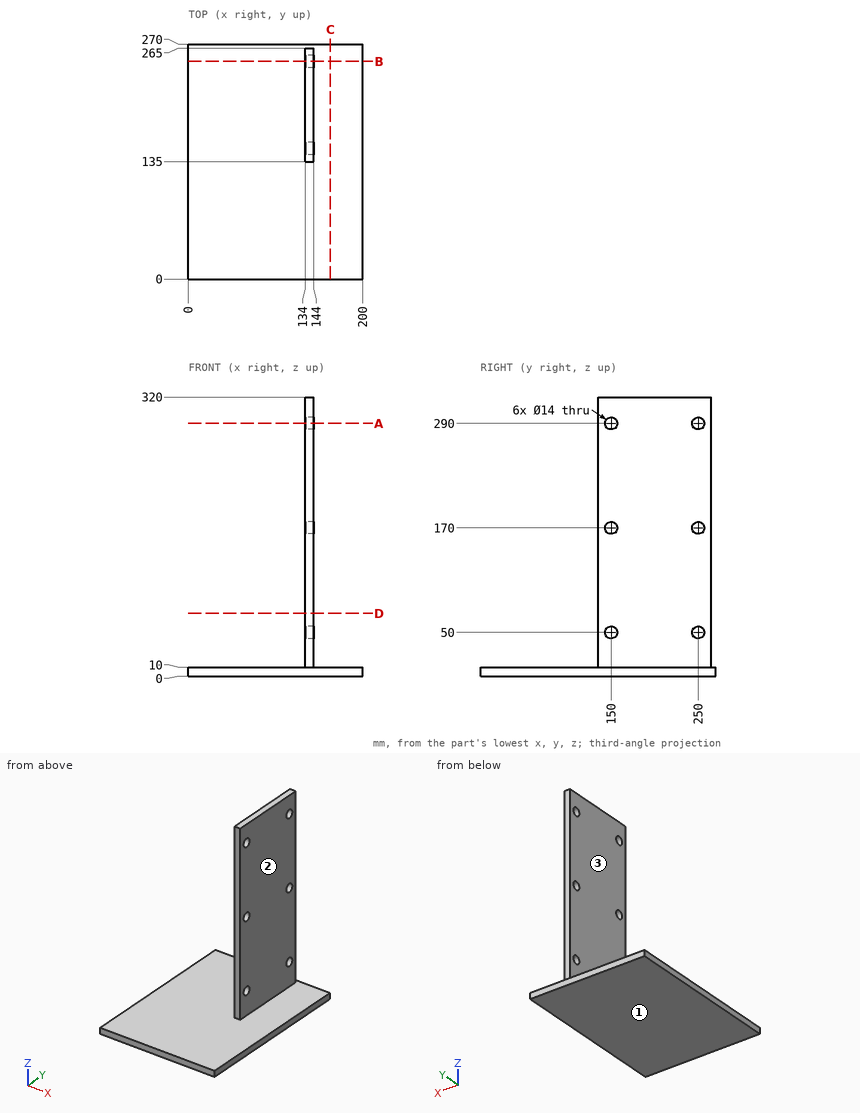
Check sheet for the drawn part. Datum: minimum x, y, z corner. Units: mm. A direction names the side the tool comes from. Round coordinates to 2 decimals unless told otherwise and drop trailing zeros. Write each loop counter-clockwise with the first axis right and the second up, starting at its lowest first coordinate (ties: lowest second). Pieces come first, ordered by that corner, then holes. Notation, with made-up numbers: (28.5, 83) -> (65.5, 83) arc R7 ccw to (65.5, 96) -> close; hole circle Ø8 at (86.25, -35). An arc over 180 degrees is marked (long way). One line per item, written item: value. Start each with the question number.
(1) Go/stop test with flat-tipped pins: pin 1 Ø8.5 at (y, z) = (150, 170) entering from -X; pin 2 Ø22.5 at (y, z) = (150, 50) entering from -X; pin 3 Ø10 at (x, y) = (64, 67) entering from +Z; pin 4 Ø8 at (x, z) = (137.5, 172.5) entering from -Y. Record where each tip stops, or that it passes through.
(2) Cross-section at A-A, the plane z = 290. Record the cut outline in (x, y).
(3) Scan lines: line 1 (Z direction, x = 139.25, y = 250); line 2 (Z direction, x = 109, y = 100); line 3 (X direction, y = 246, z = 143). Record each from-to range of solid material in increasing order. Write a range as [from, to].
(4) Access from +Z, -Z, +X, -X, +Y, -Y to the whole of each face (thin tool, end or side, straight path). Record for the marked faces 1, 2 and 3.
(5) Cross-section at D-D, the plane z = 72. Record the cut outline in (x, y).
(6) Cross-section at B-B, the plane y = 250. Record the cut outline in (x, z), and give its area (3 significant figures).
(7) Cross-section at C-C, the plane x = 163. Record the cut outline in (y, z).
Answer:
1. pin 1: through
1. pin 2: x = 134
1. pin 3: z = 10
1. pin 4: y = 135
2. outline: (134, 135) -> (144, 135) -> (144, 143) -> (134, 143) -> close; (134, 157) -> (144, 157) -> (144, 243) -> (134, 243) -> close; (134, 257) -> (144, 257) -> (144, 265) -> (134, 265) -> close
3. line 1: [0, 43], [57, 163], [177, 283], [297, 320]
3. line 2: [0, 10]
3. line 3: [134, 144]
4. face 1: -Z, +X, -X, +Y, -Y
4. face 2: +Z, +X, +Y, -Y
4. face 3: +Z, -X, +Y, -Y
5. outline: (134, 135) -> (144, 135) -> (144, 265) -> (134, 265) -> close
6. outline: (0, 0) -> (200, 0) -> (200, 10) -> (144, 10) -> (144, 43) -> (134, 43) -> (134, 10) -> (0, 10) -> close; (134, 57) -> (144, 57) -> (144, 163) -> (134, 163) -> close; (134, 177) -> (144, 177) -> (144, 283) -> (134, 283) -> close; (134, 297) -> (144, 297) -> (144, 320) -> (134, 320) -> close
6. area: 4,680 mm²
7. outline: (0, 0) -> (270, 0) -> (270, 10) -> (0, 10) -> close
